Autodesk Inventor part; units mm, degrees
ref_plane "YZ Plane" through (0, 0, 0) normal (1, 0, 0) x (0, 1, 0)
ref_plane "XZ Plane" through (0, 0, 0) normal (0, 1, 0) x (-1, 0, 0)
ref_plane "XY Plane" through (0, 0, 0) normal (0, 0, 1) x (1, 0, 0)
sketch "Sketch1" plane through (0, 0, 0) normal (0, 0, 1) x (1, 0, 0)
  line L0 (0, 0) -> (23.33, 0)
  line L1 (23.33, 0) -> (23.33, 17.54)
  line L2 (23.33, 17.54) -> (0, 17.54)
  line L3 (0, 17.54) -> (0, 0)
  dimension "d0" = 23.33
  dimension "d1" = 17.54
extrude "Extrusion1" add sketch "Sketch1" along normal blind 10.16
sketch "Sketch2" plane through (0, 0, 10.16) normal (0, 0, 1) x (1, 0, 0)
  line L0 (1.27, 16.27) -> (22.06, 16.27)
  line L1 (22.06, 16.27) -> (22.06, 1.27)
  line L2 (22.06, 1.27) -> (1.27, 1.27)
  line L3 (1.27, 1.27) -> (1.27, 16.27)
  line L4 (0, 0) -> (23.33, 0)
  line L5 (23.33, 0) -> (23.33, 17.54)
  line L6 (23.33, 17.54) -> (0, 17.54)
  line L7 (0, 17.54) -> (0, 0)
  dimension "d4" = 1.27
  dimension "d5" = 1.27
  dimension "d6" = 1.27
  dimension "d7" = 1.27
extrude "Extrusion2" cut sketch "Sketch2" against normal blind 9.16 contours L0 L1 L2 L3
sketch "Sketch3" plane through (0, 0, 1) normal (0, 0, 1) x (1, 0, 0)
  line L0 (23.33, 17.54) -> (0, 17.54) construction
  line L1 (11.665, 17.54) -> (11.665, 0) construction
  line L2 (0, 0) -> (23.33, 0) construction
  line L3 (23.33, 0) -> (23.33, 17.54) construction
  line L4 (23.33, 8.77) -> (0, 8.77) construction
  line L5 (0, 17.54) -> (0, 0) construction
  circle A0 centre (5.115, 12.52) radius 1.7
  circle A1 centre (12.96, 10.66) radius 0.5
  circle A2 centre (18.215, 12.52) radius 1.7
  line L6 (1.27, 16.27) -> (22.06, 16.27)
  dimension "d10" = 3.4
  dimension "d11" = 3.4
  dimension "d13" = 6.55
  dimension "d14" = 6.55
  dimension "d15" = 3.75
  dimension "d16" = 3.75
  dimension "d17" = 1
  dimension "d18" = 5.255
  dimension "d19" = 1.86
extrude "Extrusion3" cut sketch "Sketch3" against normal through all
sketch "Sketch4" plane through (0, 0, 0) normal (0, -1, 0) x (1, 0, 0)
  line L0 (2.54, 1.6833) -> (20.79, 1.6833)
  line L1 (20.79, 1.6833) -> (20.79, 13.6213)
  line L2 (20.79, 13.6213) -> (2.54, 13.6213)
  line L3 (2.54, 13.6213) -> (2.54, 1.6833)
  line L4 (1.27, 10.16) -> (1.27, 1)
  line L5 (22.06, 10.16) -> (22.06, 1)
  point P0 (0, 0)
  dimension "d22" = 1.27
  dimension "d23" = 1.27
  dimension "d24" = 11.938
extrude "Extrusion4" cut sketch "Sketch4" against normal up to surface (1.27 mm away)
equation "\"d5\" = d4"
equation "\"d6\" = d4"
equation "\"d7\" = d4"
equation "\"d10\" = m3_clearance"
equation "\"d11\" = d12"
equation "\"d14\" = d13"
equation "\"d16\" = d15"
equation "\"d23\" = d22"
equation "\"m3_heat_set_insert\" = 4"
equation "\"m3_clearance\" = 3.4"
equation "\"m3_heat_set_depth\" = 7"
equation "\"robot_diameter\" = 354"
equation "\"hardboard_thickness\" = 5"
equation "\"motor_centerline_height\" = 13"
properties part number "microphone_casing"
Verification items for the finished model (mm, model axes). A direction names the side the tool comes from. Give positions to 0.01 mm unless a question says otherwise; leave off trailing zeros. Loops run counter-clockwise (first coordinate to the right, second up) from the corner with the lowest first, then second, coordinate; pieces in that order, holes last.
1) Depth check by flat-ended pin: pin 1 Ø1 at (x, y) = (10, 0.5) entering from +Z; pin 2 Ø2 at (x, y) = (5.115, 12.52) entering from -Z; pin 3 Ø2.5 at (x, z) = (9.5, 6) entering from -Y. Enter the tip coordinate at first touch or a pass-through.
2) Sectioned sample at A-A, the plane y = 12.52. Enter the section's corners in (x, z) (3 decimals), then the cut area to 3 significant figures.
3) Sectioned sample at B-B, the plane x = 12.96. Enter the section's corners in (y, z).
4) Draft check along X on faces 4 (the flat face through (0, 9, 5)), 5 (the flat face through (20.79, 1, 6)), 6 (the flat face through (23.33, 9, 5)), 7 (the flat face through (11.5, 0, 0.5)). Enter one of: pulls with the +X half, pulls with the -X half, needs draft (parallel to the pull), parting line crosses it, or undercut.
5) Sectioned sample at D-D, the plane x = 20.25. Enter the section's corners in (y, z), then the cut area to 3 significant figures.
6) Sectioned sample at C-C, the plane z = 3.25. Enter the section's corners in (x, y), then the cut area to 3 significant figures.
7) Thickness scan on line 1 along X through (y, z) = (5.25, 1.75); line 2 along Y through (x, z) = (2, 9); line 3 along Z through (x, y) = (15.5, 0.75). Record the ranges inside material, lowest first.
8) Set-up check for faces 1 (the flat face through (1.27, 9, 6)), 2 (the flat face through (12, 17.54, 5)), 3 (the flat face through (2.54, 1, 6)): record each of +Z, -Z, +X, -X, +Y, -Y from which the full face is reachable in a straight line by a thin tool's end or side.
Answers:
1. pin 1: stops at z = 1.68
1. pin 2: passes through
1. pin 3: stops at y = 16.27
2. outline: (0, 0) - (3.415, 0) - (3.415, 1) - (1.27, 1) - (1.27, 10.16) - (0, 10.16) - close; (6.815, 0) - (16.515, 0) - (16.515, 1) - (6.815, 1) - close; (19.915, 0) - (23.33, 0) - (23.33, 10.16) - (22.06, 10.16) - (22.06, 1) - (19.915, 1) - close
2. area: 39.8 mm2
3. outline: (0, 0) - (10.16, 0) - (10.16, 1) - (1.27, 1) - (1.27, 1.68) - (0, 1.68) - close; (11.16, 0) - (17.54, 0) - (17.54, 10.16) - (16.27, 10.16) - (16.27, 1) - (11.16, 1) - close
4. face 4: pulls with the -X half
4. face 5: undercut
4. face 6: pulls with the +X half
4. face 7: needs draft
5. outline: (0, 0) - (17.54, 0) - (17.54, 10.16) - (16.27, 10.16) - (16.27, 1) - (1.27, 1) - (1.27, 1.68) - (0, 1.68) - close
5. area: 30.0 mm2
6. outline: (0, 0) - (2.54, 0) - (2.54, 1.27) - (1.27, 1.27) - (1.27, 16.27) - (22.06, 16.27) - (22.06, 1.27) - (20.79, 1.27) - (20.79, 0) - (23.33, 0) - (23.33, 17.54) - (0, 17.54) - close
6. area: 74.2 mm2
7. line 1: x = 0 to 1.27, 22.06 to 23.33
7. line 2: y = 0 to 1.27, 16.27 to 17.54
7. line 3: z = 0 to 1.68
8. face 1: +Z
8. face 2: +Z, -Z, +X, -X, +Y
8. face 3: +Z, -Y
